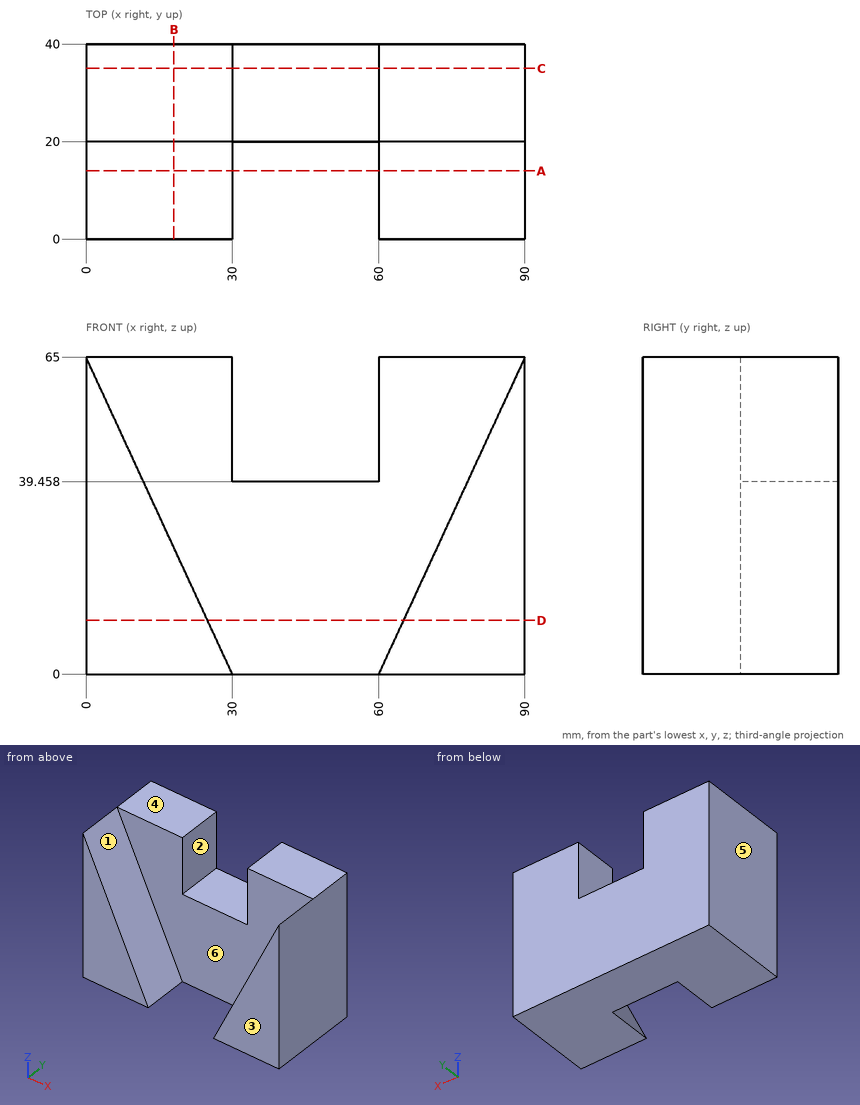
Answer from the drawing. Dimensions are ordinates in mm from the lowest x, y and z of the part. A direction names the side the tool comes from. Give positions to 0.01 mm unless a question says otherwise; leave off trailing zeros. Write each loop counter-clockwise with the first axis right and the second up, starting at its lowest first coordinate (ties: lowest second). Pieces come first, ordered by that corner, then holes. Notation, with made-up numbers: (-19, -4) - (10, -4) arc R15 cw to (10, 14) - close; hole circle Ø8 at (8, 39). An arc over 180 degrees is marked (long way). Answer in a Markdown table with one row per item. Add a question column.
Item 1: Find the intervals of material crossed by L1, parallel to X at y = 29, z = 57; L2, parallel to Z at x = 45.5, y = 27.5; L3, parallel to X at y = 4.5, z = 60, in increasing order.
Item 2: Section B-B, the plane x = 18 is taken. Write down the section's boundary in (y, z), and give its area (3 significant figures).
Item 3: Section C-C, the plane y = 35 is taken. Write down the section's boundary in (x, z), and give its area (3 significant figures).
Item 4: Section D-D, the plane z = 11 is taken. Write down the section's boundary in (x, y).
Item 5: Determine the mould class of the marked faces 4, 5 and 6 for opening direction X: pulls with the +X half, pulls with the -X half, needs draft (parallel to the pull), parting line crosses it, or undercut.
Item 6: Section A-A, the plane y = 14 is taken. Write down the section's boundary in (x, z), and give its area (3 significant figures).
Item 7: A tool of negligible diameter and unlimited length cuts with its end or side. For the marked faces 1, 2 and 3, from which of +Z, -Z, +X, -X, +Y, -Y can it reach the whole face along a straight path? Write none if from no direction.
Item 8: Flat-ended cylindrical pins translate along their axes: P1, Ø12, axis at x = 30, y = 33, coming from the -Z side; P2, Ø6, axis at x = 48.5, y = 32.5, coming from the +Z side; P3, Ø1.5, axis at x = 53, z = 31.5, coming from the -Y side. Find the tip coordinate at first contact, or state that the pin passes through.
Recorded:
| question | item | result |
|---|---|---|
| 1 | L1 | x = 0 to 30, 60 to 90 |
| 1 | L2 | z = 0 to 39.46 |
| 1 | L3 | x = 0 to 2.31, 87.69 to 90 |
| 2 | outline | (0, 0) - (40, 0) - (40, 65) - (20, 65) - (20, 26) - (0, 26) - close |
| 2 | area | 1,820 mm2 |
| 3 | outline | (0, 0) - (90, 0) - (90, 65) - (60, 65) - (60, 39.46) - (30, 39.46) - (30, 65) - (0, 65) - close |
| 3 | area | 5,080 mm2 |
| 4 | outline | (0, 0) - (24.92, 0) - (24.92, 20) - (65.08, 20) - (65.08, 0) - (90, 0) - (90, 40) - (0, 40) - close |
| 5 | face 4 | needs draft |
| 5 | face 5 | pulls with the -X half |
| 5 | face 6 | undercut |
| 6 | outline | (0, 0) - (30, 0) - (0, 65) - close; (60, 0) - (90, 0) - (90, 65) - close |
| 6 | area | 1,950 mm2 |
| 7 | face 1 | +Z, -Y |
| 7 | face 2 | +Z, +Y, -Y |
| 7 | face 3 | +Z, -Z, +X, -X, -Y |
| 8 | P1 | stops at z = 0 |
| 8 | P2 | stops at z = 39.46 |
| 8 | P3 | stops at y = 20 |
